```python
from build123d import *

# Parameters (mm, degrees)
SKETCH1_R      = 4.325
EXTRUDE1_DEPTH = 6.35


with BuildPart() as part:
    # Sketch1 → Extrude1 (new body)
    with BuildSketch(Plane(origin=(0, 0, 0), x_dir=(1, 0, 0), z_dir=(0, 1, 0))):
        with BuildLine():
            Line((0, -9.055124804), (43.550282623, -28.454685784))
            ThreePointArc((43.550282623, -28.454685784), (53.496937792, -30.809853354), (59.277793564, -22.379878865))
            ThreePointArc((59.277793564, -22.379878865), (78.989447237, -11.124841627), (84.969178064, 10.771915509))
            ThreePointArc((84.969178064, 10.771915509), (91.664608112, 20.616056931), (82.735296136, 28.490273813))
            Line((82.735296136, 28.490273813), (65.366646785, 33.285339694))
            ThreePointArc((65.366646785, 33.285339694), (46.065339232, 41.463051172), (25.302313168, 44.34613753))
            ThreePointArc((25.302313168, 44.34613753), (15.889627698, 44.942765056), (11.002555987, 36.876096458))
            Line((11.002555987, 36.876096458), (9.659067514, 34.411727615))
            ThreePointArc((9.659067514, 34.411727615), (-0.818805509, 24.364317263), (-3.587222868, 10.113978909))
            Line((-3.587222868, 10.113978909), (-4.976998188, 7.564705828))
            ThreePointArc((-4.976998188, 7.564705828), (-8.67452133, -2.597684531), (0, -9.055124804))
        make_face()
        with Locations(Location((20.103569583, 36.876096458, 0), (0, 0, 270))):  # turned: the seam where the file's is
            Circle(SKETCH1_R, mode=Mode.SUBTRACT)
        with Locations(Location((0, 0, 0), (0, 0, 270))):  # turned: the seam where the file's is
            Circle(SKETCH1_R, mode=Mode.SUBTRACT)
        with Locations(Location((50.240830228, -22.379878865, 0), (0, 0, 270))):  # turned: the seam where the file's is
            Circle(SKETCH1_R, mode=Mode.SUBTRACT)
        with Locations(Location((82.735296136, 19.490273813, 0), (0, 0, 270))):  # turned: the seam where the file's is
            Circle(SKETCH1_R, mode=Mode.SUBTRACT)
    extrude(amount=EXTRUDE1_DEPTH)


solid = part.part
```
Build history of the part. All positions in model axes, mm. Round coordinates to 2 decimals unless told otherwise and drop trailing zeros. Write each loop counter-clockwise with the first axis right and the second up, starting at its lowest first coordinate (ties: lowest second). Pieces come first, ordered by that corner, then holes. Notation, with made-up numbers: (75, 18.25) -> (128, 18.25) arc R21 cw to (128, 47.25) -> close; hole circle Ø5 at (60.5, 52.25). An arc over 180 degrees is marked (long way). Put each result on its own line as item: value.
Item 1: Slice it at D-D, the plane z = -30.5. Give the cut face in (x, y), plus the area to 3 significant figures.
Here are the results:
outline: (3.96, 0) -> (75.46, 0) -> (75.46, 6.35) -> (3.96, 6.35) -> close
area: 454 mm^2
Item 2: Wall check: probe 1 along Z at (x, y) = (79, 3); probe 2 along X at (y, z) = (4, 3.5); probe 3 along Z at (x, y) = (-1, 6). Give the ranges that are in metal, low to high. Write a range as from..to.
Here are the results:
probe 1: z = -29.52..-21.67, -17.31..11.11
probe 2: x = -8.35..-2.54, 2.54..83.27
probe 3: z = -24.03..-4.21, 4.21..9
Item 3: Two-plate mould, pull along X, no slides. Class faces 1 (the face through (41, 6.35, -8)), 2 (the face through (20.294, 3.131, -41.197)), 3 (the face through (46.349, 3.131, -41.384)): pulls with the +X half, pulls with the -X half, needs draft (parallel to the pull), parting line crosses it, or undercut.
Here are the results:
face 1: needs draft
face 2: undercut
face 3: pulls with the +X half
Item 4: Slice it at C-C, the plane x = 41. Give the cut face in (y, z).
Here are the results:
outline: (0, -42.69) -> (6.35, -42.69) -> (6.35, 27.32) -> (0, 27.32) -> close
Item 5: Slice it at A-A, the plane z = 0. Give the cut face in (x, y) (3 decimals), plus the area to 3 significant figures.
Here are the results:
outline: (-9.055, 0) -> (-4.325, 0) -> (-4.325, 6.35) -> (-9.055, 6.35) -> close; (4.325, 0) -> (84.357, 0) -> (84.357, 6.35) -> (4.325, 6.35) -> close
area: 538 mm^2
Item 6: Flat gauge pins, fed straight in: P1, Ø1.5, axis at x = 7.5, y = 4, coming from the -Z side; P2, Ø2, axis at x = 28, y = 3, coming from the -Z side; P3, Ø1, axis at y = 2.5, z = 17.5, coming from the +X side. Where does each tip first touch, or does it go through?
Here are the results:
P1: stops at z = -33.66
P2: stops at z = -44.32
P3: stops at x = 72.91
Item 7: Slice it at B-B, the plane y = 2.75. Give the cut face in (x, z) (3 decimals).
Here are the results:
outline: (-4.977, -7.565) -> (-3.587, -10.114) arc R24 ccw to (9.659, -34.412) -> (11.003, -36.876) arc R9.101 ccw to (25.302, -44.346) arc R80 ccw to (65.367, -33.285) -> (82.735, -28.49) arc R9 ccw to (84.969, -10.772) arc R29.657 ccw to (59.278, 22.38) arc R9.037 ccw to (43.55, 28.455) -> (0, 9.055) arc R9.055 ccw to start; hole circle Ø8.65 at (0, 0); hole circle Ø8.65 at (20.104, -36.876); hole circle Ø8.65 at (50.241, 22.38); hole circle Ø8.65 at (82.735, -19.49)
